The figure shows three views and two pictorial views of one solid part (mm, origin at its lowest corner). Answer the questions. A direction names the side the tool comes from. Give positions to 0.01 mm unless a question says otherwise; leave off trailing zeros. Loops run counter-clockwise (first coordinate to the right, second up) from the corner with the lowest first, then second, coordinate; pieces in that order, holes last. Notation, with made-up numbers: (17, 18.25) - (50, 18.25) arc R26 cw to (50, 50.25) - close; hole circle Ø10 at (19, 19). An arc over 180 degrees is marked (long way). Write item = value, one per line.
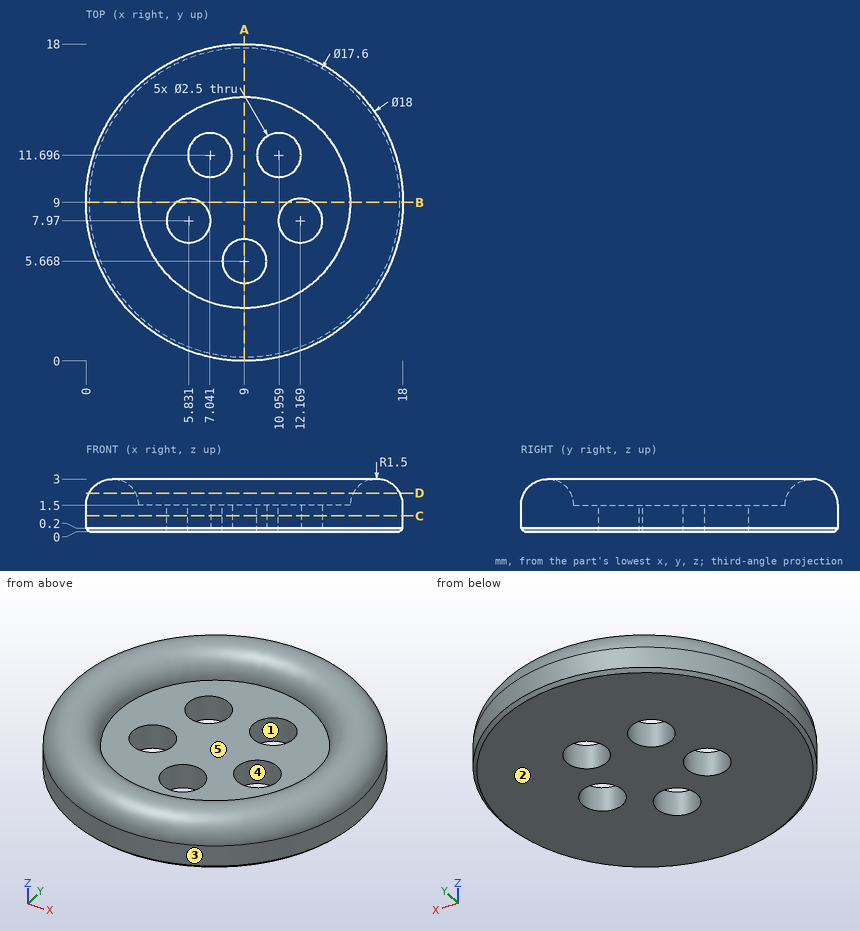
1) Each of these flat-tipped pins is pushed along its axis until it touches: P1, Ø6, axis at x = 9, y = 7.5, coming from the +Z side; P2, Ø1, axis at y = 10, z = 2.5, coming from the -X side (1 decimal); P3, Ø2, axis at x = 10.96, y = 11.7, coming from the +Z side; P4, Ø5, axis at x = 9.5, y = 15, coming from the -Z side. Where does it stop, or does it pass through?
Output:
P1 = 1.5
P2 = 0.1
P3 = through
P4 = 0
2) The mould has two halves that part along X. Classify the marked faces 1, 2 and 3: pulls with the +X half, pulls with the -X half, needs draft (parallel to the pull), parting line crosses it, or undercut.
Output:
face_1 = undercut
face_2 = needs draft
face_3 = parting line crosses it
3) Find the intervals of material crossed by probe 1 along Y at (x, z) = (9, 1.2); probe 2 along X at (y, z) = (11.75, 1.1); probe 3 along Z at (x, y) = (14.5, 9), in increasing order.
Output:
probe_1 = 0 to 4.42, 6.92 to 18
probe_2 = 0.43 to 5.79, 8.29 to 9.71, 12.21 to 17.57
probe_3 = 0 to 1.5
4) A cutting plane is placed at D-D on z = 2.2. Determine the outline of the cut face in (x, y), then the cut area to 3 significant figures.
Output:
outline = circle Ø17.65 at (9, 9); hole circle Ø12.35 at (9, 9)
area = 125 mm²
5) A cutting plane is placed at A-A on x = 9. Determine the outline of the cut face in (y, z).
Output:
outline = (0, 0.2) - (0.2, 0) - (4.42, 0) - (4.42, 1.5) - (3, 1.5) arc R1.5 ccw to (0, 1.5) - close; (6.92, 0) - (17.8, 0) - (18, 0.2) - (18, 1.5) arc R1.5 ccw to (15, 1.5) - (6.92, 1.5) - close
6) A tool of negligible diameter and unlimited length cuts with its end or side. For the marked faces 4 and 5, from which of +Z, -Z, +X, -X, +Y, -Y can it reach the whole face along a straight path? Write none if from no direction.
Output:
face_4 = +Z, -Z
face_5 = +Z
7) A cutting plane is placed at B-B on y = 9. Determine the outline of the cut face in (x, z).
Output:
outline = (0, 0.2) - (0.2, 0) - (5.12, 0) - (5.12, 1.5) - (3, 1.5) arc R1.5 ccw to (0, 1.5) - close; (6.54, 0) - (11.46, 0) - (11.46, 1.5) - (6.54, 1.5) - close; (12.88, 0) - (17.8, 0) - (18, 0.2) - (18, 1.5) arc R1.5 ccw to (15, 1.5) - (12.88, 1.5) - close
8) A cutting plane is placed at C-C on z = 0.9. Determine the outline of the cut face in (x, y), then the cut area to 3 significant figures.
Output:
outline = circle Ø18 at (9, 9); hole circle Ø2.5 at (5.83, 7.97); hole circle Ø2.5 at (7.04, 11.7); hole circle Ø2.5 at (9, 5.67); hole circle Ø2.5 at (10.96, 11.7); hole circle Ø2.5 at (12.17, 7.97)
area = 230 mm²
